from build123d import *

# Parameters (mm, degrees)
F1_DEPTH = 30


with BuildPart() as f1:
    # F0 (on Front) → F1 (new body)
    with BuildSketch(Plane.XZ):
        with BuildLine():
            Line((16.246856, 73.438403), (0, 98.65823))
            Line((0, 98.65823), (0, -51.34177))
            Line((0, -51.34177), (4, -51.34177))
            ThreePointArc((4, -51.34177), (4.181132, -48.365772), (6.370376, -46.34177))
            ThreePointArc((6.370376, -46.34177), (7.795537, -46.079272), (9.220697, -46.34177))
            Line((9.220697, -46.34177), (60.847245, -51.34177))
            Line((60.847245, -51.34177), (49.33347, -43.671459))
            ThreePointArc((49.33347, -43.671459), (47.957966, -41.291777), (48.44287, -38.58627))
            ThreePointArc((48.44287, -38.58627), (48.992071, -37.85299), (49.69371, -37.263903))
            Line((49.69371, -37.263903), (83.367956, -1.664075))
            ThreePointArc((83.367956, -1.664075), (74.347655, -4.636921), (66.910868, 1.270518))
            Line((66.910868, 1.270518), (62, 20.65823))
            Line((62, 20.65823), (42.681483, 25.834611))
            ThreePointArc((42.681483, 25.834611), (36.318117, 31.036333), (36.001559, 39.249137))
            Line((36.001559, 39.249137), (13.986726, 10.857402))
            Line((13.986726, 10.857402), (32.153903, 78.65823))
            ThreePointArc((32.153903, 78.65823), (25.612525, 71.744903), (16.246856, 73.438403))
        make_face()
        with BuildLine():
            Line((0, -51.34177), (0, 98.65823))
            Line((0, 98.65823), (-16.246856, 73.438403))
            ThreePointArc((-16.246856, 73.438403), (-25.612525, 71.744903), (-32.153903, 78.65823))
            Line((-32.153903, 78.65823), (-13.986726, 10.857402))
            Line((-13.986726, 10.857402), (-36.001559, 39.249137))
            ThreePointArc((-36.001559, 39.249137), (-36.318117, 31.036333), (-42.681483, 25.834611))
            Line((-42.681483, 25.834611), (-62, 20.65823))
            Line((-62, 20.65823), (-66.910868, 1.270518))
            ThreePointArc((-66.910868, 1.270518), (-74.347655, -4.636921), (-83.367956, -1.664075))
            Line((-83.367956, -1.664075), (-49.69371, -37.263903))
            ThreePointArc((-49.69371, -37.263903), (-48.992071, -37.85299), (-48.44287, -38.58627))
            ThreePointArc((-48.44287, -38.58627), (-47.957966, -41.291777), (-49.33347, -43.671459))
            Line((-49.33347, -43.671459), (-60.847245, -51.34177))
            Line((-60.847245, -51.34177), (-9.220697, -46.34177))
            ThreePointArc((-9.220697, -46.34177), (-5.028829, -47.190444), (-4, -51.34177))
            Line((-4, -51.34177), (-8, -81.34177))
            Line((-8, -81.34177), (0, -81.34177))
            Line((0, -81.34177), (0, -51.34177))
        make_face()
        Polygon((4, -51.34177), (0, -51.34177), (0, -81.34177), (8, -81.34177), align=None)
        with BuildLine():
            ThreePointArc((9.220697, -46.34177), (7.795537, -46.079272), (6.370376, -46.34177))
            Line((6.370376, -46.34177), (9.220697, -46.34177))
        make_face()
        with BuildLine():
            ThreePointArc((49.69371, -37.263903), (48.992071, -37.85299), (48.44287, -38.58627))
            Line((48.44287, -38.58627), (49.69371, -37.263903))
        make_face()
        with BuildLine():
            Line((-49.69371, -37.263903), (-48.44287, -38.58627))
            ThreePointArc((-48.44287, -38.58627), (-48.992071, -37.85299), (-49.69371, -37.263903))
        make_face()
    extrude(amount=F1_DEPTH)


solid = f1.part
Can you work these out from the model? Positions are in its coordinate system, mm. A direction names the side the tool comes from. Round coordinates to 2 decimals unless told otherwise and drop trailing zeros. Loops run counter-clockwise (first coordinate to the right, second up) from the corner with the lowest first, then second, coordinate; pieces in that order, holes last. Notation, with made-up numbers: (-30, 85.5) - (22, 85.5) arc R17 cw to (22, 98.5) - close; hole circle Ø4 at (-11.75, 22.25). An arc over 180 degrees is marked (long way). Write item = value, one per line. Start each with the question number.
(1) For faces 4 (the face through (-35.395, -14.79, -48.877)), 5 (the face through (-5.97, -14.79, -66.13)), 6 (the face through (8.24, -14.79, 85.87)), 7 (the face through (4.163, -14.79, -48.405)), which set-ups out of +Z, -Z, +X, -X, +Y, -Y let a thin tool reach every point of the face, with its end or its side?
(2) If we section it at A-A (z = 18.5): Please give me the cut outline in (x, y), and give its area (3 significant figures).
(3) If we section it at D-D (x = -55.5): Please give me the cut outline in (y, z).
(4) If we mould it in two halves opening along Z, with no side actions, what happens to faces 1 (the face through (64.49, -14.79, 10.83)), 2 (the face through (0, -15, -81.342)), 3 (the face through (25.148, -14.79, 25.252))? For each: released by +Z, released by -Z, zero draft, split by the parting line, or undercut.
(5) If we section it at B-B (x = 52): Please give me the cut outline in (y, z).
(6) For P1, Ø12, axis at x = -13, z = -56.5, coming from the +Y side; P2, Ø6, axis at x = -42, z = -11.5, coming from the +Y side; P3, Ø10, axis at x = 32, y = -19, coming from the -Z side; P4, Ø12, axis at y = -22, z = -31.5, coming from the +X side, each with a flat end and sliding along its axis, tell me the tip position at first contact or that it passes through.
(7) If I drill on probe 1 along X at (y, z) = (-5.25, 34); probe 2 along X at (y, z) = (-7.75, 12); probe 3 along Z at (x, y) = (-51.5, -5.5), over which ranges is the centre line in solid material (lowest first)? Write a range as [from, to].
Ans:
q1.face_4 = -Z, +Y, -Y
q1.face_5 = -X, +Y, -Y
q1.face_6 = +Z, +Y, -Y
q1.face_7 = +Y, -Y
q2.outline = (-62.55, -30) - (-19.91, -30) - (-19.91, 0) - (-62.55, 0) - close; (-16.03, -30) - (16.03, -30) - (16.03, 0) - (-16.03, 0) - close; (19.91, -30) - (62.55, -30) - (62.55, 0) - (19.91, 0) - close
q2.area = 3,520 mm²
q3.outline = (-30, -50.82) - (0, -50.82) - (0, -47.78) - (-30, -47.78) - close; (-30, -31.13) - (0, -31.13) - (0, 22.4) - (-30, 22.4) - close
q4.face_1 = released by +Z
q4.face_2 = released by -Z
q4.face_3 = undercut
q5.outline = (-30, -50.48) - (0, -50.48) - (0, -45.45) - (-30, -45.45) - close; (-30, -34.83) - (0, -34.83) - (0, 23.34) - (-30, 23.34) - close
q6.P1 = through
q6.P2 = 0
q6.P3 = -49.03
q6.P4 = 60.82
q7.probe_1 = [-35.38, -31.93], [-20.19, 20.19], [31.93, 35.38]
q7.probe_2 = [-64.19, -14.87], [-14.29, 14.29], [14.87, 64.19]
q7.probe_3 = [-50.44, -45.11], [-35.35, 23.47]
